```python
from build123d import *

# Parameters (mm, degrees)
BOSS_EXTRUDE1_DEPTH = 20
SKETCH2_R           = 3
CUT_EXTRUDE1_DEPTH  = 5.5
SKETCH3_R           = 3
CUT_EXTRUDE2_DEPTH  = 5.5
BOSS_EXTRUDE2_DEPTH = 2
BOSS_EXTRUDE3_DEPTH = 2


with BuildPart() as part:
    # Sketch1 → Boss-Extrude1 (new body, symmetric)
    with BuildSketch(Plane(origin=(0, 0, 0), x_dir=(0, 0, -1), z_dir=(1, 0, 0))):
        Polygon((0, 0), (0, 30), (-4.5, 30), (-4.5, 4.5), (-30, 4.5), (-30, 0), align=None)
    extrude(amount=BOSS_EXTRUDE1_DEPTH, both=True)

    # Sketch2 → Cut-Extrude1 (cut, through all)
    with BuildSketch(Plane.XY.offset(4.5)):
        with Locations((-10, 18)):
            Circle(SKETCH2_R)
        with Locations((10, 18)):
            Circle(SKETCH2_R)
    extrude(amount=-CUT_EXTRUDE1_DEPTH, mode=Mode.SUBTRACT)

    # Sketch3 → Cut-Extrude2 (cut, through all)
    with BuildSketch(Plane(origin=(0, 4.5, 0), x_dir=(1, 0, 0), z_dir=(0, 1, 0))):
        with Locations((-10, -10)):
            Circle(SKETCH3_R)
        with Locations((-10, -18)):
            Circle(SKETCH3_R)
        with Locations((10, -10)):
            Circle(SKETCH3_R)
        with Locations((10, -18)):
            Circle(SKETCH3_R)
    extrude(amount=-CUT_EXTRUDE2_DEPTH, mode=Mode.SUBTRACT)

    # Sketch4 → Boss-Extrude2 (add)
    with BuildSketch(Plane(origin=(20, 0, 0), x_dir=(0, 0, -1), z_dir=(1, 0, 0))):
        Polygon((0, 0), (0, 30), (-4.5, 30), (-30, 4.5), (-30, 0), align=None)
    extrude(amount=-BOSS_EXTRUDE2_DEPTH)

    # Sketch5 → Boss-Extrude3 (add)
    with BuildSketch(Plane.ZY.offset(20)):
        Polygon((30, 4.5), (4.5, 30), (4.5, 4.5), align=None)
    extrude(amount=-BOSS_EXTRUDE3_DEPTH)


solid = part.part
```
Here's how the part is built. I have some questions about the finished solid (model axes, mm). A direction names the side the tool comes from. Coordinates: 2 decimals unless noted, no trailing zeros. Order: outer loops, then holes, each group sorted by start corner. A loop starts at its lowest first (then second) coordinate and runs counter-clockwise, first axis right, second up. Notation, with made-up numbers: M 23,-23.5 L 80,-23.5 A19 ccw 80,4.5 Z; hole C 46.5,-23.75 d9. An arc over 180 degrees is marked long. Answer as a JSON object with one key per item and string values. Group by question number.
(1) I need wall thicknesses on probe 1 along X at (y, z) = (3.05, 18); probe 2 along Z at (x, y) = (10, 2.5); probe 3 along X at (y, z) = (13.5, 18.5). Which ranges of each line are inside material? Lowest first, please.
(2) Suppose I cut it at A-A, the plane x = -10. Please give me the cut outline in (y, z), then the cut area to 3 significant figures.
(3) Suppose I cut it at D-D, the plane y = 13.75. Please give me the cut outline in (x, z).
(4) Suppose I cut it at C-C, the plane z = 10. Please give me the cut outline in (x, y).
(5) Which directions (+Z, -Z, +X, -X, +Y, -Y) give clear straight access to the entire face, cutting with the end or side of a thin tool? Please do faces 5 (the face through (0, 30, 2)), 6 (the face through (18, 12, 12)).
(6) If we mould it in two halves opening along X, with no side actions, what happens to faces 1 (the face through (-20, 12, 11)), 2 (the face through (-19, 17.1, 17.4)), 3 (the face through (20, 12, 12)), 4 (the face through (11.384, 2.282, 20.662))? For each: released by +X, released by -X, zero draft, split by the parting line, or undercut.
(7) Suppose I cut it at B-B, the plane y = 18. Please give me the cut outline in (x, z).
(8) For pin 1 (7.5 mm diameter, centred on x = -6, y = 20.5, fed in from +Z); pin 2 (7.5 mm diameter, centred on x = 0.5, z = 16, fed in from +Y), each with a flat end and sliding along its axis, tell me the tip position at first contact or that it passes through.
Values found:
{
 "1": {"probe 1": "x = -20 to -13, -7 to 7, 13 to 20", "probe 2": "z = 0 to 7, 13 to 15, 21 to 30", "probe 3": "x = -20 to -18, 18 to 20"},
 "2": {"outline": "M 0,0 L 15,0 L 15,4.5 L 4.5,4.5 L 4.5,7 L 0,7 Z; M 0,13 L 4.5,13 L 4.5,15 L 0,15 Z; M 0,21 L 4.5,21 L 4.5,30 L 0,30 Z; M 21,0 L 30,0 L 30,4.5 L 21,4.5 Z", "area": "169 mm^2"},
 "3": {"outline": "M -20,0 L 20,0 L 20,20.75 L 18,20.75 L 18,4.5 L -18,4.5 L -18,20.75 L -20,20.75 Z"},
 "4": {"outline": "M -20,0 L -13,0 L -13,4.5 L -18,4.5 L -18,24.5 L -20,24.5 Z; M -7,0 L 7,0 L 7,4.5 L -7,4.5 Z; M 13,0 L 20,0 L 20,24.5 L 18,24.5 L 18,4.5 L 13,4.5 Z"},
 "5": {"face 5": "+Z, -Z, +X, -X, +Y", "face 6": "+Z, +Y"},
 "6": {"face 1": "released by -X", "face 2": "zero draft", "face 3": "released by +X", "face 4": "undercut"},
 "7": {"outline": "M -20,0 L -13,0 L -13,4.5 L -18,4.5 L -18,16.5 L -20,16.5 Z; M -7,0 L 7,0 L 7,4.5 L -7,4.5 Z; M 13,0 L 20,0 L 20,16.5 L 18,16.5 L 18,4.5 L 13,4.5 Z"},
 "8": {"pin 1": "stops at z = 4.5", "pin 2": "stops at y = 4.5"}
}
